Check sheet for the drawn part. Datum: minimum x, y, z corner. Units: mm. A direction names the side the tool comes from. Coordinates: 2 decimals unless noted, no trailing zeros. Loops run counter-clockwise (first coordinate to the right, second up) from the corner with the lowest first, then second, coordinate; pieces in that order, holes last. Notation, with made-up numbers: M 4,27 L 18,27 A11 ccw 18,31 Z; hole C 41.5,63 d10. An arc over 180 degrees is marked long. Answer as CSV lines item,"result". Start each with the question number.
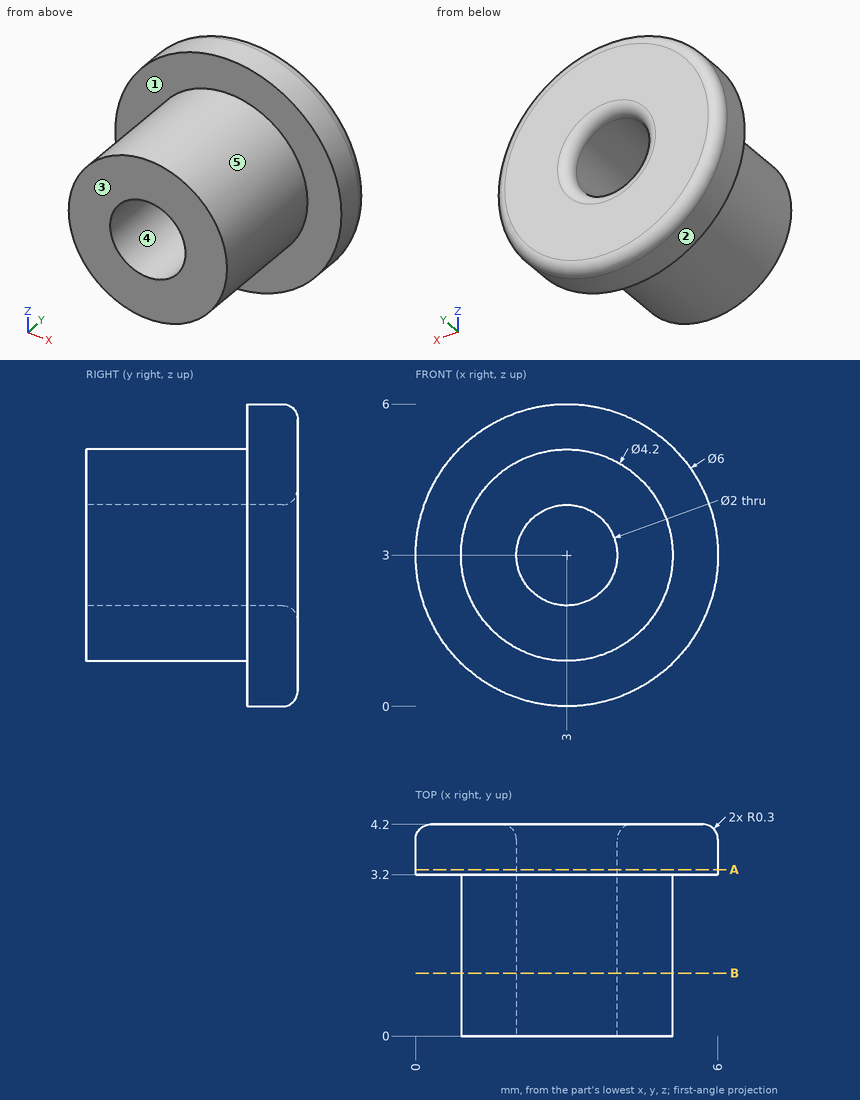
Item 1: Set-up check for the marked faces 1 and 2: record each of +Z, -Z, +X, -X, +Y, -Y from which the full face is reachable in a straight line by a thin tool's end or side.
Item 2: Material ranges on line 1 (Z direction, x = 3, y = 1.1); line 2 (Y direction, x = 3, z = 0.5); line 3 (X direction, y = 1.95, z = 3.5), recorded low to high. Write a range as from..to.
Item 3: Sectioned sample at A-A, the plane y = 3.3. Record the boundary of the cut face in (x, z), and give its area (3 significant figures).
Item 4: Go/stop test with flat-tipped pins: pin 1 (2 mm diameter, centred on x = 1, y = 2, fed in from +Z); pin 2 (1.6 mm diameter, centred on x = 3, z = 3, fed in from +Y); pin 3 (2 mm diameter, centred on y = 2.5, z = 4.5, fed in from +X). Record where each tip stops, or that it passes through.
Item 5: Release check for a two-part mould opening along Z. For the marked faces 3, 4 and 5 record: released by +Z, released by -Z, zero draft, split by the parting line, or undercut.
Item 6: Sectioned sample at B-B, the plane y = 1.25. Record the boundary of the cut face in (x, z), and give its area (3 significant figures).
Reply:
1,face 1,"-Y"
1,face 2,"+Y, -Y"
2,line 1,"0.9..2, 4..5.1"
2,line 2,"3.2..4.2"
2,line 3,"0.96..2.13, 3.87..5.04"
3,outline,"C 3,3 d6; hole C 3,3 d2"
3,area,"25.1 mm²"
4,pin 1,"z = 4.85"
4,pin 2,"through"
4,pin 3,"x = 5.9"
5,face 3,"zero draft"
5,face 4,"undercut"
5,face 5,"split by the parting line"
6,outline,"C 3,3 d4.2; hole C 3,3 d2"
6,area,"10.7 mm²"
